Design review of the part built by this model. Coordinates are the model's own, in mm. Face numbers are marked on the shaded views. A direction names the side the tool comes from. Coordinates: 2 decimals unless noted, no trailing zeros. Write each loop counter-clockwise with the first axis right and the second up, starting at its lowest first coordinate (ties: lowest second). Pieces come first, ordered by that corner, then holes.
Q1. Take a section at A-A, the plane x = 21. Write out the cut boundary in (y, z), plus the area to 3 significant figures.
Q2. For the marked faces 4 and 5, list the 3-axis set-ups (+Z, -Z, +X, -X, +Y, -Y) from which the entire face can be reached by the end or side of a thin tool; tool diameter is ignored.
Q3. The part is to be moulded in two halves that separate along Z. For the marked faces 1, 2 and 3, say which applies: released by +Z, released by -Z, zero draft, split by the parting line, or undercut.
Q4. For pin 1 Ø2 at (y, z) = (10, 8.5) entering from +X; pin 2 Ø2 at (x, z) = (11, 7) entering from +Y; pin 3 Ø2.5 at (x, z) = (21, 5) entering from -Y, all flat-tipped, find the tip position at first contact; note any pin that passes through.
Q5. For L1, parallel to Z at x = 21, y = 1.2; L2, parallel to X at y = 19.5, z = 8, list the stretches that pass through material, from the lowest coordinate up.
Q6. Take a section at D-D, the plane z = 8.75. Write out the cut boundary in (x, y).
Q7. Take a section at C-C, the plane z = 5. Write out the cut boundary in (x, y), plus the area to 3 significant figures.
from build123d import *

# Parameters (mm, degrees)
PAD_DEPTH       = 10
SKETCH001_R     = 1.5
POCKET_DEPTH    = 5
SKETCH002_R     = 1.5
POCKET001_DEPTH = 5


with BuildPart() as part:
    # Sketch → Pad (new body)
    with BuildSketch(Plane.XY):
        Polygon((0, 0), (0, 26), (3, 26), (3, 3), (26, 3), (26, 0), align=None)
    extrude(amount=PAD_DEPTH)

    # Sketch001 (on Face6 of Pad) → Pocket (cut)
    with BuildSketch(Plane.XZ):
        with Locations((21, 5)):
            Circle(SKETCH001_R)
    extrude(amount=-POCKET_DEPTH, mode=Mode.SUBTRACT)

    # Sketch002 (on Face1 of Pocket) → Pocket001 (cut)
    with BuildSketch(Plane(origin=(0, 0, 0), x_dir=(0, -1, 0), z_dir=(-1, 0, 0))):
        with Locations((-21, 5)):
            Circle(SKETCH002_R)
    extrude(amount=-POCKET001_DEPTH, mode=Mode.SUBTRACT)


solid = part.part
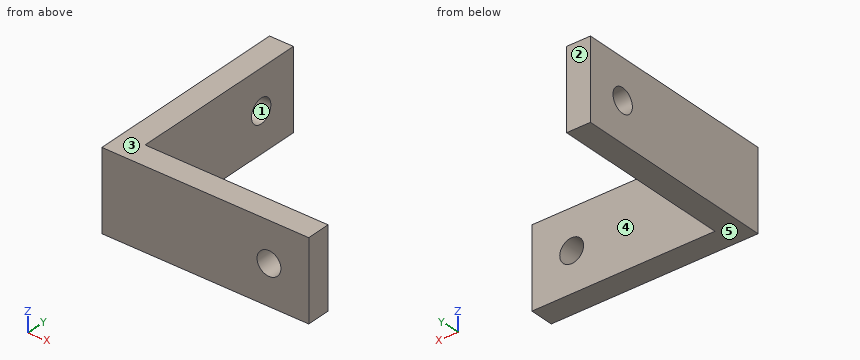
Responses:
1. outline: (0, 0) - (3, 0) - (3, 3.5) - (0, 3.5) - close; (0, 6.5) - (3, 6.5) - (3, 10) - (0, 10) - close
1. area: 21.0 mm2
2. face 4: +Z, -Z, +X, +Y
2. face 5: -Z, +X, -X, +Y, -Y
3. face 1: undercut
3. face 2: zero draft
3. face 3: released by +Z
4. pin 1: stops at x = 3
4. pin 2: stops at y = 3
4. pin 3: passes through
5. L1: z = 0 to 3.5, 6.5 to 10
5. L2: x = 0 to 3
6. outline: (0, 0) - (26, 0) - (26, 3) - (3, 3) - (3, 26) - (0, 26) - close
7. outline: (0, 0) - (19.5, 0) - (19.5, 3) - (3, 3) - (3, 19.5) - (0, 19.5) - close; (0, 22.5) - (3, 22.5) - (3, 26) - (0, 26) - close; (22.5, 0) - (26, 0) - (26, 3) - (22.5, 3) - close
7. area: 129 mm2
